from build123d import *

# Parameters (mm, degrees)
BOSS_EXTRUDE1_DEPTH = 3
CUT_EXTRUDE1_REACH  = 66.915
SKETCH2_R           = 4.25
SKETCH2_R_2         = 1.05
SKETCH3_R           = 1.9
CUT_EXTRUDE2_DEPTH  = 1
BOSS_EXTRUDE2_DEPTH = 29
BOSS_EXTRUDE4_DEPTH = 3
CUT_EXTRUDE3_REACH  = 184.811
SKETCH8_R           = 1.05
SKETCH9_R           = 1.9
CUT_EXTRUDE4_DEPTH  = 1
CUT_EXTRUDE5_REACH  = 185.098
BOSS_EXTRUDE8_REACH = 186.206
SKETCH16_W          = 3.2
SKETCH16_H          = 2
CUT_EXTRUDE6_DEPTH  = 186.123769408
CUT_EXTRUDE7_REACH  = 186.206
SKETCH17_W          = 7
SKETCH17_H          = 11


with BuildPart() as part:
    # Sketch1 → Boss-Extrude1 (new body)
    with BuildSketch(Plane.XY):
        with BuildLine():
            Line((25, 29), (48.666332079, 25.373055569))
            ThreePointArc((48.666332079, 25.373055569), (58, 14.5), (48.666332079, 3.626944431))
            Line((48.666332079, 3.626944431), (25, 0))
            Line((25, 0), (0, 0))
            Line((0, 0), (0, 29))
            Line((0, 29), (25, 29))
        make_face()
    extrude(amount=-BOSS_EXTRUDE1_DEPTH)

    # Sketch2 → Cut-Extrude1 (cut, up to next)
    with BuildSketch(Plane.XY, mode=Mode.PRIVATE) as cut_extrude1_sk1:
        with Locations((47, 14.5)):
            Circle(SKETCH2_R)
    cut_extrude1_tool1 = extrude(cut_extrude1_sk1.sketch, amount=-CUT_EXTRUDE1_REACH, mode=Mode.PRIVATE) & part.part
    # Sketch2 → Cut-Extrude1 (cut, up to next)
    with BuildSketch(Plane.XY, mode=Mode.PRIVATE) as cut_extrude1_sk2:
        with Locations((47, 22.5)):
            Circle(SKETCH2_R_2)
    cut_extrude1_tool2 = extrude(cut_extrude1_sk2.sketch, amount=-CUT_EXTRUDE1_REACH, mode=Mode.PRIVATE) & part.part
    # Sketch2 → Cut-Extrude1 (cut, up to next)
    with BuildSketch(Plane.XY, mode=Mode.PRIVATE) as cut_extrude1_sk3:
        with Locations((55, 14.5)):
            Circle(SKETCH2_R_2)
    cut_extrude1_tool3 = extrude(cut_extrude1_sk3.sketch, amount=-CUT_EXTRUDE1_REACH, mode=Mode.PRIVATE) & part.part
    # Sketch2 → Cut-Extrude1 (cut, up to next)
    with BuildSketch(Plane.XY, mode=Mode.PRIVATE) as cut_extrude1_sk4:
        with Locations((47, 6.5)):
            Circle(SKETCH2_R_2)
    cut_extrude1_tool4 = extrude(cut_extrude1_sk4.sketch, amount=-CUT_EXTRUDE1_REACH, mode=Mode.PRIVATE) & part.part
    # Sketch2 → Cut-Extrude1 (cut, up to next)
    with BuildSketch(Plane.XY, mode=Mode.PRIVATE) as cut_extrude1_sk5:
        with Locations((39, 14.5)):
            Circle(SKETCH2_R_2)
    cut_extrude1_tool5 = extrude(cut_extrude1_sk5.sketch, amount=-CUT_EXTRUDE1_REACH, mode=Mode.PRIVATE) & part.part
    add(cut_extrude1_tool1.solids().sort_by_distance((47, 14.5, 0))[0], mode=Mode.SUBTRACT)
    add(cut_extrude1_tool2.solids().sort_by_distance((47, 22.5, 0))[0], mode=Mode.SUBTRACT)
    add(cut_extrude1_tool3.solids().sort_by_distance((55, 14.5, 0))[0], mode=Mode.SUBTRACT)
    add(cut_extrude1_tool4.solids().sort_by_distance((47, 6.5, 0))[0], mode=Mode.SUBTRACT)
    add(cut_extrude1_tool5.solids().sort_by_distance((39, 14.5, 0))[0], mode=Mode.SUBTRACT)

    # Sketch3 → Cut-Extrude2 (cut)
    with BuildSketch(Plane.XY):
        with Locations((47, 22.5)):
            Circle(SKETCH3_R)
        with Locations((55, 14.5)):
            Circle(SKETCH3_R)
        with Locations((47, 6.5)):
            Circle(SKETCH3_R)
        with Locations((39, 14.5)):
            Circle(SKETCH3_R)
    extrude(amount=-CUT_EXTRUDE2_DEPTH, mode=Mode.SUBTRACT)

    # Sketch4 → Boss-Extrude2 (add)
    with BuildSketch(Plane(origin=(0, 29, 0), x_dir=(1, 0, 0), z_dir=(0, 1, 0))):
        Polygon((0, 3), (0, 0), (-30, 10), (-130, 10), (-160, 5), (-160, 8), (-130, 13), (-30, 13), align=None)
    extrude(amount=-BOSS_EXTRUDE2_DEPTH)

    # Sketch7 → Boss-Extrude4 (add)
    with BuildSketch(Plane.XY.offset(-5)):
        Polygon((-160, 29), (-164.7, 33.7), (-179.5, 33.7), (-179.5, 25), (-166, 25), (-166, 4), (-179.5, 4), (-179.5, -4.7), (-164.7, -4.7), (-160, 0), align=None)
    extrude(amount=-BOSS_EXTRUDE4_DEPTH)

    # Sketch8 → Cut-Extrude3 (cut, up to next)
    with BuildSketch(Plane.XY.offset(-5), mode=Mode.PRIVATE) as cut_extrude3_sk1:
        with Locations((-176.25, 28)):
            Circle(SKETCH8_R)
    cut_extrude3_tool1 = extrude(cut_extrude3_sk1.sketch, amount=-CUT_EXTRUDE3_REACH, mode=Mode.PRIVATE) & part.part
    # Sketch8 → Cut-Extrude3 (cut, up to next)
    with BuildSketch(Plane.XY.offset(-5), mode=Mode.PRIVATE) as cut_extrude3_sk2:
        with Locations((-168.25, 28)):
            Circle(SKETCH8_R)
    cut_extrude3_tool2 = extrude(cut_extrude3_sk2.sketch, amount=-CUT_EXTRUDE3_REACH, mode=Mode.PRIVATE) & part.part
    # Sketch8 → Cut-Extrude3 (cut, up to next)
    with BuildSketch(Plane.XY.offset(-5), mode=Mode.PRIVATE) as cut_extrude3_sk3:
        with Locations((-163, 22.5)):
            Circle(SKETCH8_R)
    cut_extrude3_tool3 = extrude(cut_extrude3_sk3.sketch, amount=-CUT_EXTRUDE3_REACH, mode=Mode.PRIVATE) & part.part
    # Sketch8 → Cut-Extrude3 (cut, up to next)
    with BuildSketch(Plane.XY.offset(-5), mode=Mode.PRIVATE) as cut_extrude3_sk4:
        with Locations((-163, 6.5)):
            Circle(SKETCH8_R)
    cut_extrude3_tool4 = extrude(cut_extrude3_sk4.sketch, amount=-CUT_EXTRUDE3_REACH, mode=Mode.PRIVATE) & part.part
    # Sketch8 → Cut-Extrude3 (cut, up to next)
    with BuildSketch(Plane.XY.offset(-5), mode=Mode.PRIVATE) as cut_extrude3_sk5:
        with Locations((-168.25, 1)):
            Circle(SKETCH8_R)
    cut_extrude3_tool5 = extrude(cut_extrude3_sk5.sketch, amount=-CUT_EXTRUDE3_REACH, mode=Mode.PRIVATE) & part.part
    # Sketch8 → Cut-Extrude3 (cut, up to next)
    with BuildSketch(Plane.XY.offset(-5), mode=Mode.PRIVATE) as cut_extrude3_sk6:
        with Locations((-176.25, 1)):
            Circle(SKETCH8_R)
    cut_extrude3_tool6 = extrude(cut_extrude3_sk6.sketch, amount=-CUT_EXTRUDE3_REACH, mode=Mode.PRIVATE) & part.part
    add(cut_extrude3_tool1.solids().sort_by_distance((-176.25, 28, -5))[0], mode=Mode.SUBTRACT)
    add(cut_extrude3_tool2.solids().sort_by_distance((-168.25, 28, -5))[0], mode=Mode.SUBTRACT)
    add(cut_extrude3_tool3.solids().sort_by_distance((-163, 22.5, -5))[0], mode=Mode.SUBTRACT)
    add(cut_extrude3_tool4.solids().sort_by_distance((-163, 6.5, -5))[0], mode=Mode.SUBTRACT)
    add(cut_extrude3_tool5.solids().sort_by_distance((-168.25, 1, -5))[0], mode=Mode.SUBTRACT)
    add(cut_extrude3_tool6.solids().sort_by_distance((-176.25, 1, -5))[0], mode=Mode.SUBTRACT)

    # Sketch9 → Cut-Extrude4 (cut)
    with BuildSketch(Plane.XY.offset(-5)):
        with Locations((-176.25, 28)):
            Circle(SKETCH9_R)
        with Locations((-168.25, 28)):
            Circle(SKETCH9_R)
        with Locations((-163, 22.5)):
            Circle(SKETCH9_R)
        with Locations((-163, 6.5)):
            Circle(SKETCH9_R)
        with Locations((-168.25, 1)):
            Circle(SKETCH9_R)
        with Locations((-176.25, 1)):
            Circle(SKETCH9_R)
    extrude(amount=-CUT_EXTRUDE4_DEPTH, mode=Mode.SUBTRACT)

    # Cut-Extrude5: up to this face of the body (flat: up to its plane)
    cut_extrude5_end = Plane(part.part.faces().sort_by_distance((-80, 14.5, -13))[0])
    # Sketch11 → Cut-Extrude5 (cut, up to the picked face)
    with BuildSketch(Plane.XY, mode=Mode.PRIVATE) as cut_extrude5_sk1:
        Polygon((0, 0), (-30, 2), (-130, 2), (-160, 0), align=None)
    cut_extrude5_tool1 = split(extrude(cut_extrude5_sk1.sketch, amount=-CUT_EXTRUDE5_REACH, mode=Mode.PRIVATE), bisect_by=cut_extrude5_end, keep=Keep.BOTH, mode=Mode.PRIVATE)
    # Sketch11 → Cut-Extrude5 (cut, up to the picked face)
    with BuildSketch(Plane.XY, mode=Mode.PRIVATE) as cut_extrude5_sk2:
        Polygon((0, 29), (-30, 27), (-130, 27), (-160, 29), align=None)
    cut_extrude5_tool2 = split(extrude(cut_extrude5_sk2.sketch, amount=-CUT_EXTRUDE5_REACH, mode=Mode.PRIVATE), bisect_by=cut_extrude5_end, keep=Keep.BOTH, mode=Mode.PRIVATE)
    add(cut_extrude5_tool1.solids().sort_by(Axis((-80, 0.923077, 0), (0, 0, -1)))[0], mode=Mode.SUBTRACT)
    add(cut_extrude5_tool2.solids().sort_by(Axis((-80, 28.076923, 0), (0, 0, -1)))[0], mode=Mode.SUBTRACT)

    # Sketch14 → Boss-Extrude8 (add, up to next)
    with BuildSketch(Plane.XY.offset(-24), mode=Mode.PRIVATE) as boss_extrude8_sk1:
        Polygon((-179.5, 33.7), (-179.5, 30.7), (-164.7, 30.7), (-160, 26), (-130, 24), (-30, 24), (0, 26), (25, 26), (25, 29), (0, 29), (-30, 27), (-130, 27), (-160, 29), (-164.7, 33.7), align=None)
    boss_extrude8_tool1 = extrude(boss_extrude8_sk1.sketch, amount=BOSS_EXTRUDE8_REACH, mode=Mode.PRIVATE) - part.part
    boss_extrude8 = boss_extrude8_tool1.solids().sort_by_distance((-77.25, 26.622763, -24))[0]
    add(boss_extrude8)

    # Mirror1: Boss-Extrude8 across plane
    add(boss_extrude8.mirror(Plane.ZX.offset(14.5)))

    # Sketch16 → Cut-Extrude6 (cut, through all)
    with BuildSketch(Plane(origin=(0, 33.7, 0), x_dir=(1, 0, 0), z_dir=(0, 1, 0))):
        with Locations((-172.9, 20)):
            Rectangle(SKETCH16_W, SKETCH16_H)
        with Locations((-80, 20)):
            Rectangle(SKETCH16_W, SKETCH16_H)
        with Locations((10.6, 20)):
            Rectangle(SKETCH16_W, SKETCH16_H)
    extrude(amount=-CUT_EXTRUDE6_DEPTH, mode=Mode.SUBTRACT)

    # Sketch17 → Cut-Extrude7 (cut, up to next)
    with BuildSketch(Plane.XY, mode=Mode.PRIVATE) as cut_extrude7_sk1:
        with Locations((-151.5, 14.5)):
            Rectangle(SKETCH17_W, SKETCH17_H)
    cut_extrude7_tool1 = extrude(cut_extrude7_sk1.sketch, amount=-CUT_EXTRUDE7_REACH, mode=Mode.PRIVATE) & part.part
    # Sketch17 → Cut-Extrude7 (cut, up to next)
    with BuildSketch(Plane.XY, mode=Mode.PRIVATE) as cut_extrude7_sk2:
        with Locations((16.5, 14.5)):
            Rectangle(SKETCH17_W, SKETCH17_H)
    cut_extrude7_tool2 = extrude(cut_extrude7_sk2.sketch, amount=-CUT_EXTRUDE7_REACH, mode=Mode.PRIVATE) & part.part
    add(cut_extrude7_tool1.solids().sort_by_distance((-151.5, 14.5, 0))[0], mode=Mode.SUBTRACT)
    add(cut_extrude7_tool2.solids().sort_by_distance((16.5, 14.5, 0))[0], mode=Mode.SUBTRACT)


solid = part.part
The model under review builds one solid part; all positions refer to its coordinate system, in mm. A direction names the side the tool comes from. Give positions to 0.01 mm unless a question says otherwise; leave off trailing zeros. Write each loop counter-clockwise with the first axis right and the second up, starting at its lowest first coordinate (ties: lowest second). Pieces come first, ordered by that corner, then holes. Notation, with made-up numbers: M 56.5,27.25 L 73.5,27.25 A31 ccw 73.5,62.25 Z; hole C -40,10.5 d6. An arc over 180 degrees is marked long. One line per question, with ' | ' between items. Start each with the question number.
Item 1: Wall thickness on line 1 (Y direction, x = -168.25, z = -7.6); line 2 (Y direction, x = -162.5, z = -6.75); line 3 (Y direction, x = -150, z = -21.75): over which ranges is each line inside the solid? List them lowest first. Write a range as from..to.
Item 2: We need section B-B on x = -4. Write out the cut boundary in (y, z), plus the area to 3 significant figures.
Item 3: Draft analysis for pull direction X (two halves, no side actions). For faces 4 (the flat face through (13, 29, -12)), 5 (the cylindrical face through (-169.65, 29.284, -5.493)), 6 (the flat face through (-15, 25, -16)), state which applies: released by +X, released by -X, zero draft, split by the parting line, or undercut.
Item 4: For pin 1 (4 mm diameter, centred on y = 20, z = -3, fed in from +X); pin 2 (10 mm diameter, centred on y = 26.5, z = -20, fed in from -X); pin 3 (5 mm diameter, centred on x = -176.25, y = 28, fed in from -Z); pin 4 (3.5 mm diameter, centred on x = -62.5, z = -17, fed in from -Y), all flat-tipped, find the tip position at first contact; note any pin that passes through.
Item 5: For faces 1 (the flat face through (-15, 15, -8)), 2 (the flat face through (-80.7, 5, -18.6)), 3 (the cylindrical face through (-164.4, 23.784, -5.493)), list the 3-axis set-ups (+Z, -Z, +X, -X, +Y, -Y) from which the entire face can be reached by the end or side of a thin tool; tool diameter is ignored.
Item 6: We need section A-A on x = -101.5. Write out the cut boundary in (y, z).
Results found:
1) line 1: y = -4.7..-0.05, 2.05..4, 25..26.95, 29.05..33.7 | line 2: y = -2.5..5.58, 7.42..21.58, 23.42..31.5 | line 3: y = 0.67..3.67, 25.33..28.33
2) outline: M 0.27,-24 L 3.27,-24 L 3.27,-4.33 L 25.73,-4.33 L 25.73,-24 L 28.73,-24 L 28.73,-1.33 L 0.27,-1.33 Z | area: 203 mm2
3) face 4: zero draft | face 5: undercut | face 6: released by +X
4) pin 1: stops at x = 57.43 | pin 2: stops at x = -179.5 | pin 3: stops at z = -8 | pin 4: stops at y = 2
5) face 1: -Z, +X | face 2: -Z, +X, -X | face 3: +Z
6) outline: M 2,-24 L 5,-24 L 5,-13 L 24,-13 L 24,-24 L 27,-24 L 27,-10 L 2,-10 Z
